CAD build for the part. Positions are in the model's coordinates, mm. Give positions to 0.01 mm unless a question says otherwise; leave off trailing zeros. Loops run counter-clockwise (first coordinate to the right, second up) from the corner with the lowest first, then second, coordinate; pieces in that order, holes last. Notation, with made-up numbers: M 86.5,-7 L 95.5,-7 A23 ccw 95.5,3 Z; hole C 10,-24.75 d4. An arc over 180 degrees is marked long. Answer as CSV lines item,"result".
from build123d import *

# Parameters (mm, degrees)
SKETCH2_R           = 1
BOSS_EXTRUDE1_DEPTH = 3.175


with BuildPart() as part:
    # Sketch2 → Boss-Extrude1 (new body)
    with BuildSketch(Plane(origin=(0, 0, 0), x_dir=(1, 0, 0), z_dir=(0, 1, 0))):
        with BuildLine():
            Line((-179.386599243, -46.577112428), (-152.973973641, -46.577112428))
            ThreePointArc((-152.973973641, -46.577112428), (-151.696632976, -46.495196962), (-150.440219102, -46.250792593))
            Line((-150.440219102, -46.250792593), (-132.369306257, -41.517613837))
            ThreePointArc((-132.369306257, -41.517613837), (-129.228271572, -40.906602915), (-126.03491991, -40.70181425))
            Line((-126.03491991, -40.70181425), (-75.228071606, -40.70181425))
            ThreePointArc((-75.228071606, -40.70181425), (-65.278674057, -38.051439272), (-57.966239939, -30.802763092))
            Line((-57.966239939, -30.802763092), (-53.58197864, -23.310359981))
            ThreePointArc((-53.58197864, -23.310359981), (-51.642560943, -18.685572059), (-50.980718724, -13.714458582))
            Line((-50.980718724, -13.714458582), (-50.980718724, -11.480720615))
            ThreePointArc((-50.980718724, -11.480720615), (-55.872159917, 3.284056393), (-68.611443065, 12.207928979))
            Line((-68.611443065, 12.207928979), (-77.287357217, 14.807803777))
            add(Edge.make_bspline(
                [(-77.287357217, 14.807803777), (-78.60290824, 15.260617984), (-80.496334385, 15.662389675), (-81.330596094, 15.796728052), (-81.912447463, 15.872382986), (-82.202137874, 15.903094978), (-82.558274171, 15.939367788), (-82.869941903, 15.961449205)],
                knots=[0.680418275, 0.680418275, 0.680418275, 0.836668275, 0.899168275, 0.935139496, 0.961668275, 0.966389496, 1, 1, 1], degree=2))
            Line((-82.869941903, 15.961449205), (-168.585599211, 22.03433695))
            ThreePointArc((-168.585599211, 22.03433695), (-169.908476001, 22.040340453), (-171.220569819, 21.871672567))
            ThreePointArc((-171.220569819, 21.871672567), (-177.816509337, 19.029235729), (-182.649967908, 13.716652219))
            add(Edge.make_bspline(
                [(-182.649967908, 13.716652219), (-184.020157032, 11.266604381), (-186.59553254, 6.270980952), (-189.973739026, -1.442317999), (-192.87751868, -9.367305357), (-194.495666875, -14.743968327), (-195.233463462, -17.45250711)],
                knots=[0.255798806, 0.255798806, 0.255798806, 0.255798806, 0.412929873, 0.570060941, 0.727192008, 0.884323076, 0.884323076, 0.884323076, 0.884323076], degree=3))
            ThreePointArc((-195.233463462, -17.45250711), (-196.09568693, -21.651142502), (-196.548238057, -25.913438355))
            ThreePointArc((-196.548238057, -25.913438355), (-192.037135811, -39.625265598), (-179.386599243, -46.577112428))
        make_face()
        with Locations(Location((-66.522348751, -35.882736145, 0), (0, 0, 270))):
            Circle(SKETCH2_R, mode=Mode.SUBTRACT)
        with Locations(Location((-57.877663419, 1.791422578, 0), (0, 0, 270))):
            Circle(SKETCH2_R, mode=Mode.SUBTRACT)
        with Locations(Location((-105.433568659, 14.889534132, 0), (0, 0, 270))):
            Circle(SKETCH2_R, mode=Mode.SUBTRACT)
        with Locations(Location((-176.36445576, 16.994158234, 0), (0, 0, 270))):
            Circle(SKETCH2_R, mode=Mode.SUBTRACT)
        with Locations(Location((-190.160816791, -37.970957718, 0), (0, 0, 270))):
            Circle(SKETCH2_R, mode=Mode.SUBTRACT)
        with Locations(Location((-126.03491991, -38.20181425, 0), (0, 0, 270))):
            Circle(SKETCH2_R, mode=Mode.SUBTRACT)
    extrude(amount=BOSS_EXTRUDE1_DEPTH)


solid = part.part
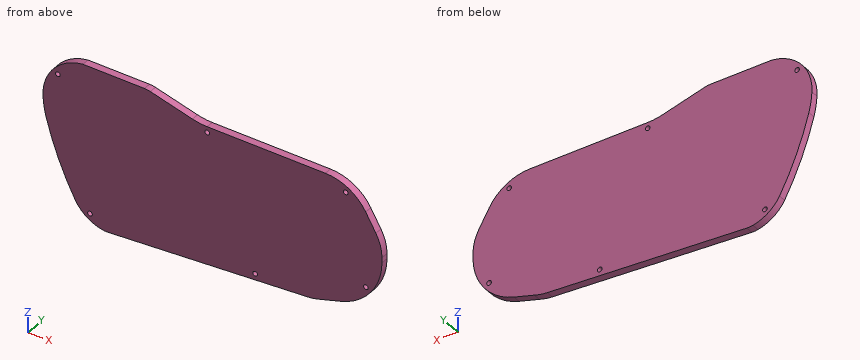
1) Drill centre lines: line 1 (Z direction, x = -106, y = 1.95); line 2 (Z direction, x = -136, y = 1.85); line 3 (Z direction, x = -170, y = 0.8). Where is each one in solid material? Low to high. Write a range as from..to.
Answer below:
line 1,"z = -17.6..-15.71, -14.07..40.7"
line 2,"z = -19.73..42.47"
line 3,"z = -22.03..46.58"
2) Band-saw the part on A-A on x = -113.5. Give the cut face in (y, z) (3 decimals).
Answer below:
outline,"M 0,-18.132 L 3.175,-18.132 L 3.175,40.702 L 0,40.702 Z"
3) Flat gauge pins, fed straight in: pin 1 (1 mm diameter, centred on x = -113.5, y = 1.5, fed in from -Z); pin 2 (1 mm diameter, centred on x = -109, y = 1, fed in from +Z). Where does each tip first touch, or does it go through?
Answer below:
pin 1,"stops at z = -18.17"
pin 2,"stops at z = 40.7"
4) Band-saw the part on C-C on y = 0.85. Give the number of separate pieces and of enclosed holes in the cut face, and give its area (3 significant figures).
Answer below:
separate pieces,"1"
enclosed holes,"6"
area,"8,180 mm^2"
5) Band-saw the part on B-B on z = 33. Give the cut face in (x, y) (3 decimals), and give its area (3 significant figures).
Answer below:
outline,"M -195.658,0 L -59.456,0 L -59.456,3.175 L -195.658,3.175 Z"
area,"432 mm^2"
